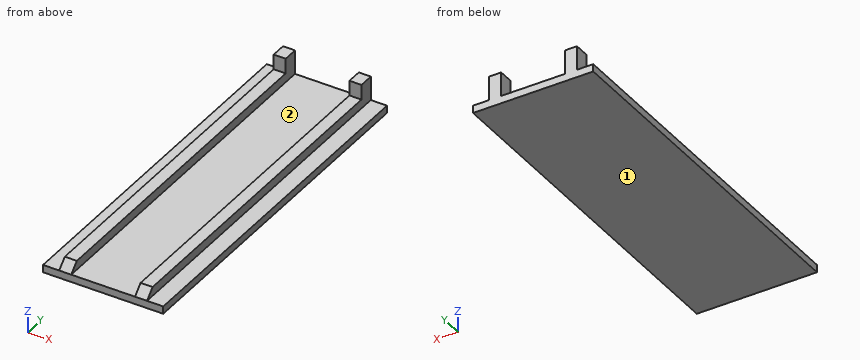
```python
from build123d import *

# Parameters (mm, degrees)
F0_W     = 40
F0_H     = 120
F1_DEPTH = 2.5
F2_W     = 4
F2_H     = 120
F3_DEPTH = 3
F4_SIZE  = 3
F5_W     = 4
F5_H     = 5
F6_DEPTH = 5


with BuildPart() as f1:
    # F0 (on Top) → F1 (new body)
    with BuildSketch(Plane.XY):
        Rectangle(F0_W, F0_H)
    extrude(amount=F1_DEPTH)

    # F2 (on face) → F3 (join)
    with BuildSketch(Plane.XY.offset(2.5)):
        with Locations((-12.606392, 0)):
            Rectangle(F2_W, F2_H)
        with Locations((12.606392, 0)):
            Rectangle(F2_W, F2_H)
    extrude(amount=F3_DEPTH)

    # F4
    f4_edges = [f1.edges().sort_by_distance(p)[0] for p in [
        (-12.606392, -60, 5.5),
        (12.606392, -60, 5.5),
    ]]
    chamfer(f4_edges, length=F4_SIZE)

    # F5 (on face) → F6 (join)
    with BuildSketch(Plane.XY.offset(5.5)):
        with Locations((12.606392, 57.5)):
            Rectangle(F5_W, F5_H)
        with Locations((-12.606392, 57.5)):
            Rectangle(F5_W, F5_H)
    extrude(amount=F6_DEPTH)


solid = f1.part
```
Model file for the job. Use its own axes, mm. Face numbers are marked on the shaded views. A direction names the side the tool comes from. Coordinates: 2 decimals unless noted, no trailing zeros. Loops run counter-clockwise (first coordinate to the right, second up) from the corner with the lowest first, then second, coordinate; pieces in that order, holes last. Notation, with made-up numbers: (85.5, -1) - (138.5, -1) arc R19 ccw to (138.5, 13) - close; hole circle Ø10 at (-7.5, 70.25). An arc over 180 degrees is marked (long way). Write item = value, one per line. Start each with the question number.
Item 1: Wall check: probe 1 along X at (y, z) = (-42.5, 4.75); probe 2 along Z at (x, y) = (13, 48.5); probe 3 along Y at (x, z) = (14.5, 7.75). Give the ranges that are in metal, low to high. Write a range as [from, to].
Item 2: Drop flat-ended pins along their axis: pin 1 Ø23.5 at (x, y) = (-1, -2) entering from +Z; pin 2 Ø4.5 at (x, y) = (18, -1.5) entering from +Z; pin 3 Ø1.5 at (y, z) = (0, 4.5) entering from +X. Give the stop position or say it passes through.
Item 3: 3-axis set-ups, long thin cutter, end or side, ignore diameter. For the marked faces 1 and 2: which of +Z, -Z, +X, -X, +Y, -Y reach the whole face in a straight line?
Item 4: Saw through at C-C, the plane x = 12.5. List the corners of the cut face in (y, z), then the cut area to 4 significant figures.
Item 5: Saw through at B-B, the plane y = 0. List the corners of the cut face in (x, z).
Item 6: Saw through at A-A, the plane z = 4. List the corners of the cut face in (x, y), then the cut area to 3 significant figures.
Item 7: Saw through at D-D, the plane x = 5. List the corners of the cut face in (y, z).
Answers:
q1.probe_1 = [-14.61, -10.61], [10.61, 14.61]
q1.probe_2 = [0, 5.5]
q1.probe_3 = [55, 60]
q2.pin_1 = 5.5
q2.pin_2 = 2.5
q2.pin_3 = 14.61
q3.face_1 = -Z, +X, -X, +Y, -Y
q3.face_2 = +Z, +Y, -Y
q4.outline = (-60, 0) - (60, 0) - (60, 10.5) - (55, 10.5) - (55, 5.5) - (-57, 5.5) - (-60, 2.5) - close
q4.area = 680.5 mm2
q5.outline = (-20, 0) - (20, 0) - (20, 2.5) - (14.61, 2.5) - (14.61, 5.5) - (10.61, 5.5) - (10.61, 2.5) - (-10.61, 2.5) - (-10.61, 5.5) - (-14.61, 5.5) - (-14.61, 2.5) - (-20, 2.5) - close
q6.outline = (-14.61, -58.5) - (-10.61, -58.5) - (-10.61, 60) - (-14.61, 60) - close; (10.61, -58.5) - (14.61, -58.5) - (14.61, 60) - (10.61, 60) - close
q6.area = 948 mm2
q7.outline = (-60, 0) - (60, 0) - (60, 2.5) - (-60, 2.5) - close
